```python
from build123d import *

# Parameters (mm, degrees)
SKETCH1_W           = 200
SKETCH1_H           = 200
SKETCH1_R           = 2
SKETCH1_W_2         = 15
SKETCH1_H_2         = 4
BOSS_EXTRUDE1_DEPTH = 4


with BuildPart() as part:
    # Sketch1 → Boss-Extrude1 (new body)
    with BuildSketch(Plane(origin=(0, 0, 0), x_dir=(1, 0, 0), z_dir=(0, 1, 0))):
        with Locations((100, -100)):
            Rectangle(SKETCH1_W, SKETCH1_H)
        with Locations((100, -61.75)):
            Circle(SKETCH1_R, mode=Mode.SUBTRACT)
        with Locations((100, -51.75)):
            Circle(SKETCH1_R, mode=Mode.SUBTRACT)
        with Locations((100, -148.25)):
            Circle(SKETCH1_R, mode=Mode.SUBTRACT)
        with Locations((100, -138.25)):
            Circle(SKETCH1_R, mode=Mode.SUBTRACT)
        with Locations((61.75, -100)):
            Circle(SKETCH1_R, mode=Mode.SUBTRACT)
        with Locations((51.75, -100)):
            Circle(SKETCH1_R, mode=Mode.SUBTRACT)
        with Locations((138.25, -100)):
            Circle(SKETCH1_R, mode=Mode.SUBTRACT)
        with Locations((148.25, -100)):
            Circle(SKETCH1_R, mode=Mode.SUBTRACT)
        with Locations((30, -12)):
            Rectangle(SKETCH1_W_2, SKETCH1_H_2, mode=Mode.SUBTRACT)
        with Locations((65, -12)):
            Rectangle(SKETCH1_W_2, SKETCH1_H_2, mode=Mode.SUBTRACT)
        with Locations((100, -12)):
            Rectangle(SKETCH1_W_2, SKETCH1_H_2, mode=Mode.SUBTRACT)
        with Locations((135, -12)):
            Rectangle(SKETCH1_W_2, SKETCH1_H_2, mode=Mode.SUBTRACT)
        with Locations((170, -12)):
            Rectangle(SKETCH1_W_2, SKETCH1_H_2, mode=Mode.SUBTRACT)
        with Locations((170, -188)):
            Rectangle(SKETCH1_W_2, SKETCH1_H_2, mode=Mode.SUBTRACT)
        with Locations((135, -188)):
            Rectangle(SKETCH1_W_2, SKETCH1_H_2, mode=Mode.SUBTRACT)
        with Locations((100, -188)):
            Rectangle(SKETCH1_W_2, SKETCH1_H_2, mode=Mode.SUBTRACT)
        with Locations((65, -188)):
            Rectangle(SKETCH1_W_2, SKETCH1_H_2, mode=Mode.SUBTRACT)
        with Locations((30, -188)):
            Rectangle(SKETCH1_W_2, SKETCH1_H_2, mode=Mode.SUBTRACT)
    extrude(amount=BOSS_EXTRUDE1_DEPTH)


solid = part.part
```
The model under review builds one solid part; all positions refer to its coordinate system, in mm. Give positions to 0.01 mm unless a question says otherwise; leave off trailing zeros. Write each loop counter-clockwise with the first axis right and the second up, starting at its lowest first coordinate (ties: lowest second). Pieces come first, ordered by that corner, then holes. Notation, with made-up numbers: (12.5, 66) -> (50.5, 66) arc R23 cw to (50.5, 98) -> close; hole circle Ø1 at (-5.5, 40.5). An arc over 180 degrees is marked (long way). Put each result on its own line as item: value.
(1) We need section A-A, the plane x = 105. Give the boundary of the cut face in (y, z), and give its area (3 significant figures).
Results are:
outline: (0, 0) -> (4, 0) -> (4, 10) -> (0, 10) -> close; (0, 14) -> (4, 14) -> (4, 186) -> (0, 186) -> close; (0, 190) -> (4, 190) -> (4, 200) -> (0, 200) -> close
area: 768 mm²
(2) To check wall thickness, follow probe 1 along X at (y, z) = (1.9, 100); probe 2 along Z at (x, y) = (136, 1.95); probe 3 along Z at (x, y) = (138.25, 2.45). State the ranges of each line that lie inside material, in increasing order. Write a range as from..to.
Results are:
probe 1: 0..49.75, 53.75..59.75, 63.75..136.25, 140.25..146.25, 150.25..200
probe 2: 0..10, 14..186, 190..200
probe 3: 0..10, 14..98, 102..186, 190..200
(3) We need section B-B, the plane y = 2.5. State how many separate pieces and enclosed holes the cut face has, and give its area (3 significant figures).
Results are:
separate pieces: 1
enclosed holes: 18
area: 39,300 mm²
